Input: part model. Units: mm. Frame: model coordinates. Face numbers are marked on the shaded views. A direction names the side the tool comes from. Round coordinates to 2 decimals unless told otherwise and drop trailing zeros. Order: outer loops, then holes, each group sorted by start corner. A loop starts at its lowest first (then second) coordinate and runs counter-clockwise, first axis right, second up. Notation, with made-up numbers: (-39.75, 29) -> (-4.75, 29) arc R19 cw to (-4.75, 43) -> close; hole circle Ø11 at (74.25, 16). An arc over 180 degrees is marked (long way). Use a Markdown table: item, result.
Autodesk Inventor part; units mm, degrees
ref_plane "Belt Plane" through (0, 31, 8) normal (0, 0, 1) x (1, 0, 0)
ref_plane "YZ Plane" through (0, 0, 0) normal (1, 0, 0) x (0, 1, 0)
ref_plane "XZ Plane" through (0, 0, 0) normal (0, 1, 0) x (-1, 0, 0)
sketch "Main Sketch" plane through (0, 0, 0) normal (1, 0, 0) x (0, 1, 0)
  line L0 (0, 28) -> (42, 28)
  line L1 (42, 28) -> (42, 12.8615)
  line L2 (42, 12.8615) -> (31, 9.4984)
  line L3 (31, 9.4984) -> (31, 6.5016)
  line L4 (31, 6.5016) -> (42, 3.1385)
  line L5 (42, 3.1385) -> (42, 0)
  line L6 (42, 0) -> (0, 0)
  line L7 (40, 12.25) -> (40, 3.75) construction
  line L8 (31, 8) -> (40, 8) construction
  line L9 (42, 12.8615) -> (42, 3.1385)
  line L10 (0, -5.6) -> (0, 33.6)
  line L11 (0, 0) -> (0, 28)
  line L12 (36, 0) -> (36, 3.5)
  line L13 (36, 3.5) -> (15, 3.5)
  line L14 (15, 3.5) -> (15, 0)
  line L15 (36, 28) -> (36, 24.5)
  line L16 (36, 24.5) -> (15, 24.5)
  line L17 (15, 24.5) -> (15, 28)
  dimension "d0" = 8.5
  dimension "d1" = 34
  dimension "d2" = 2
  dimension "d6" = 28
  dimension "d21" = 80
  dimension "d25" = 11
  dimension "d27" = 8
  dimension "d35" = 6
  dimension "d36" = 15
  dimension "d37" = 3.5
ref_plane "Belt Plane" through (0, 31, 8) normal (0, 0, 1) x (1, 0, 0)
revolve "Body" add sketch "Main Sketch" angle 360 about axis through (0, 0, -10) along (0, 0, 1) contours L0 L17 L16 L15 L1 L2 L3 L4 L5 L6 L12 L13 L14 L10 | L9 L4 L3 L2
revolve "Groove" cut sketch "Main Sketch" angle 360 about axis through (0, 0, -10) along (0, 0, 1) contours L9 L4 L3 L2
fillet "Fillet External" [suppressed]
fillet "Fillet Internal" [suppressed]
pattern_linear "Groove Pattern" count 2 spacing 12 along (0, 0, 1) of "Groove"
sketch "Sketch2" plane through (0, 0, 0) normal (0, 0, -1) x (-1, 0, 0)
  circle A0 centre (0, 0) radius 42
hole "Hole1" at (0, 0, 0) direction (0, 0, 1) diameter 6.6 end through all counterbore diameter 18 counterbore depth 23
equation "\"d0\" = da_Bw"
equation "\"d1\" = da_Alfa"
equation "\"d2\" = da_c"
equation "\"d21\" = da_Dw"
equation "\"d25\" = da_Hd"
equation "\"d27\" = da_Se"
equation "\"da_r1\" = 0"
equation "\"da_r2\" = 0"
equation "\"d18\" = da_Sg"
equation "\"d5\" = da_Se"
equation "\"da_Bw\" = 8.5"
equation "\"da_Alfa\" = 34deg"
equation "\"da_c\" = 2"
equation "\"da_Dw\" = 80"
equation "\"da_Hd\" = 11"
equation "\"da_Se\" = 8"
equation "\"da_Sg\" = 12"
properties part number "PWTR-0096" material "Stainless Steel"
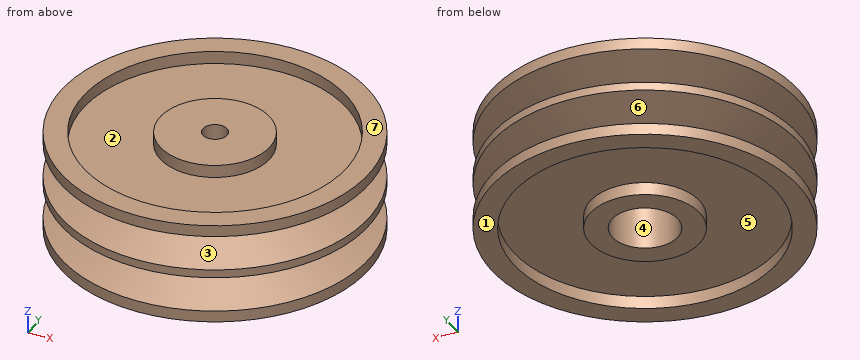
1) Cut plane B-B on y = 34. Count the separate pieces of the cut face and the enclosed holes in it, and give its area (3 significant figures).
Results found:
| item | result |
|---|---|
| separate pieces | 3 |
| enclosed holes | 0 |
| area | 571 mm² |
2) Cut plane A-A on z = 16.75. Return loops of the section in (x, y), and give its area (3 significant figures).
Results found:
| item | result |
|---|---|
| outline | circle Ø73.46 at (0, 0); hole circle Ø18 at (0, 0) |
| area | 3,980 mm² |
3) Set-up query: the marked faces 5, 6 and 7. Return all of +Z, -Z, +X, -X, +Y, -Y with unobstructed straight access to the full face (end or side cutting, diameter ignored); none if empty.
Results found:
| item | result |
|---|---|
| face 5 | -Z |
| face 6 | none |
| face 7 | +Z, +X, -X, +Y, -Y |
4) Line query: L1, parallel to Y at x = 0, z = 27.35; L2, parallel to Z at x = -26, y = 18.5. Output: solid intervals per line, ascending. Write a range as [from, to].
Results found:
| item | result |
|---|---|
| L1 | y = [-42, -36], [-15, -3.3], [3.3, 15], [36, 42] |
| L2 | z = [3.5, 6.22], [9.78, 18.22], [21.78, 24.5] |
5) Pin query (flat end, axial travel): pin 1 Ø5.5 at (x, y) = (0, 0) entering from +Z; pin 2 Ø5 at (x, y) = (18.5, 14.5) entering from +Z; pin 3 Ø4 at (x, z) = (9.5, 3) entering from +Y; pin 4 Ø10 at (x, z) = (-18.5, 24.5) entering from +Y. Return the tip coordinate at first contact, or that it passes through.
Results found:
| item | result |
|---|---|
| pin 1 | passes through |
| pin 2 | stops at z = 24.5 |
| pin 3 | stops at y = 41.32 |
| pin 4 | stops at y = 39.77 |
6) Pull-direction query (Z, two-part tool) for the marked faces 1, 2, 3 and 4; classes: +Z half, -Z half, draft (parallel to the pull), parting line (faces both ways), or undercut.
Results found:
| item | result |
|---|---|
| face 1 | -Z half |
| face 2 | +Z half |
| face 3 | undercut |
| face 4 | draft |
